Autodesk Inventor part; units mm, degrees
ref_plane "YZ Plane" through (0, 0, 0) normal (1, 0, 0) x (0, 1, 0)
ref_plane "XZ Plane" through (0, 0, 0) normal (0, 1, 0) x (-1, 0, 0)
ref_plane "XY Plane" through (0, 0, 0) normal (0, 0, 1) x (1, 0, 0)
sketch "Sketch1" plane through (0, 0, 0) normal (0, 0, 1) x (1, 0, 0)
  line L0 (0, 0) -> (15.24, 0)
  line L1 (21.2852, 0) -> (21.2852, 12.5984)
  line L2 (21.2852, 12.5984) -> (0, 12.5984)
  line L3 (0, 12.5984) -> (0, 0)
  line L4 (15.24, 0) -> (15.24, -15.621)
  line L5 (15.24, -15.621) -> (21.2852, -15.621)
  line L6 (21.2852, -15.621) -> (21.2852, 0)
  line L7 (0, 0) -> (15.24, 0)
  dimension "d0" = 21.2852
  dimension "d1" = 12.5984
  dimension "d2" = 6.0452
  dimension "d3" = 15.621
extrude "Extrusion1" add sketch "Sketch1" along normal blind 1.4986
sketch "Sketch2" plane through (0, 0, 1.4986) normal (0, 0, 1) x (1, 0, 0)
  circle A0 centre (4.572, 6.5532) radius 1.9558
  line L0 (21.2852, 12.5984) -> (0, 12.5984)
  line L1 (0, 12.5984) -> (0, 0)
  circle A1 centre (18.2626, 6.5532) radius 1.9558
  dimension "d6" = 3.9116
  dimension "d7" = 6.0452
  dimension "d8" = 4.572
  dimension "d11" = 13.6906
extrude "Extrusion2" cut sketch "Sketch2" against normal blind 25.4
sketch "Sketch3" plane through (0, 0, 1.4986) normal (0, 0, 1) x (1, 0, 0)
  circle A0 centre (18.2626, -11.6332) radius 1.4478
  line L0 (15.24, -15.621) -> (21.2852, -15.621)
  line L1 (15.24, 0) -> (15.24, -15.621)
  circle A1 centre (18.2626, -7.6708) radius 1.4478
  line L2 (16.8148, -7.6708) -> (18.2626, -7.6708)
  line L3 (19.7104, -11.6332) -> (17.1196, -11.6332)
  point P0 (0, 0)
  dimension "d18" = 2.8956
  dimension "d19" = 3.9878
  dimension "d20" = 3.0226
  dimension "d26" = 3.9624
extrude "Extrusion4" cut sketch "Sketch3" against normal blind 25.4
sketch "Sketch6" plane through (0, 0, 1.4986) normal (0, 0, 1) x (1, 0, 0)
  circle A0 centre (18.2626, -7.6708) radius 1.4478
  circle A1 centre (18.2626, -11.6332) radius 1.4478
  line L0 (16.8148, -7.6708) -> (19.7104, -7.6708)
  line L1 (19.7104, -7.6708) -> (19.7104, -11.6332)
  line L2 (19.7104, -11.6332) -> (16.8148, -11.6332)
  line L3 (16.8148, -11.6332) -> (16.8148, -7.6708)
  point P0 (0, 0)
extrude "Extrusion5" cut sketch "Sketch6" against normal blind 25.4 contours L1 A1 L3 A0 | A0 L0 | L2 A1 picked at (18.2044, -8.1499) picked at (18.4337, -11.182)
sketch "Sketch17" plane through (0, 0, 0) normal (0, 0, -1) x (-1, 0, 0)
  line L0 (-21.2852, -15.621) -> (-21.2852, 12.5984)
  line L1 (-21.2852, 0) -> (-15.349, 0)
  point P0 (0, 0)
bend part "Bend Part3" radius 1.4986 angle 90 line through (21.2852, 0, 0) along (-1, 0, 0) centre toward (0, 0, -1) moving side (0, -1, 0) both sides no
equation "\"BendRadius\" = Thickness"
equation "\"BendReliefWidth\" = Thickness"
equation "\"BendReliefDepth\" = 0.5 * Thickness"
equation "\"CornerReliefSize\" = 4 * Thickness"
equation "\"MinimumRemnant\" = 2 * Thickness"
equation "\"TransitionRadius\" = BendRadius"
equation "\"JacobiRadiusSize\" = Thickness"
equation "\"GapSize\" = Thickness"
properties part number "dsub37bracket_redraw"
CAD build for the part. Positions are in the model's coordinates, mm. A direction names the side the tool comes from. Coordinates: 2 decimals unless noted, no trailing zeros. Loops run counter-clockwise (first coordinate to the right, second up) from the corner with the lowest first, then second, coordinate; pieces in that order, holes last. Notation, with made-up numbers: (-23.5, 82) - (15.5, 82) arc R17 ccw to (15.5, 106) - close; hole circle Ø4 at (-8.5, -12.5). An arc over 180 degrees is marked (long way). Write item = value, one per line. Start each with the question number.
Q1. Pull direction Z, two halves, no side cores. Call faces 5 (the cylindrical face through (18.231, -2.258, -12.225)), 6 (the flat face through (0, 6, 1)), 7 (the flat face through (10, 6, 0)), 8 (the flat face through (10, 6, 1.499)): pulls with the +Z half, pulls with the -Z half, needs draft (parallel to the pull), parting line crosses it, or undercut.
Q2. Cut at C-C, the plane y = 5.75. List the corners of the cut face in (x, z), then the cut area to 3 significant figures.
Q3. Cut at A-A, the plane z = -8. List the corners of the cut face in (x, y).
Q4. Flat gauge pins, fed straight in: pin 1 Ø5 at (x, y) = (4.57, 6.55) entering from -Z; pin 2 Ø5 at (x, z) = (8, -2) entering from -Y; pin 3 Ø1.5 at (y, z) = (-1, -6) entering from -X. Where does each tip first touch, or does it go through?
Q5. Drill centre lines: L1, parallel to Z at x = 16, y = 1; L2, parallel to Y at x = 19.5, z = -13.25; L3, parallel to X at y = 7, z = 0.75. Where is each one in solid material? Low to high.
Q6. Cut at B-B, the plane x = 18.5. List the corners of the cut face in (y, z).
Q7. Cut at D-D, the plane x = 3.75. List the corners of the cut face in (y, z), then the cut area to 3 significant figures.
Q8. Which spindle directions (+Z, -Z, +X, -X, +Y, -Y) get a long thin tool onto all of the face, cutting with end or side? Do faces 1 (the flat face through (16, -2.997, -8)), 2 (the cylindrical face through (18.294, -2.258, -5.368)), 3 (the flat face through (8, 0, 1)), 4 (the flat face through (16, -1.499, -8)). Say none if no direction does.
Computed:
q1.face_5 = undercut
q1.face_6 = needs draft
q1.face_7 = pulls with the -Z half
q1.face_8 = pulls with the +Z half
q2.outline = (0, 0) - (2.79, 0) - (2.79, 1.5) - (0, 1.5) - close; (6.36, 0) - (16.48, 0) - (16.48, 1.5) - (6.36, 1.5) - close; (20.05, 0) - (21.29, 0) - (21.29, 1.5) - (20.05, 1.5) - close
q2.area = 21.2 mm²
q3.outline = (15.24, -3) - (16.81, -3) - (16.81, -1.5) - (15.24, -1.5) - close; (19.71, -3) - (21.29, -3) - (21.29, -1.5) - (19.71, -1.5) - close
q4.pin_1 = 0
q4.pin_2 = 0
q4.pin_3 = 15.24
q5.L1 = 0 to 1.5
q5.L2 = -3 to -1.5
q5.L3 = 0 to 2.67, 6.48 to 16.36, 20.17 to 21.29
q6.outline = (-3, -14.77) - (-1.5, -14.77) - (-1.5, -12.21) - (-3, -12.21) - close; (-3, -5.39) - (-1.5, -5.39) - (-1.5, -1.5) arc R1.5 cw to (0, 0) - (4.61, 0) - (4.61, 1.5) - (0, 1.5) arc R3 ccw to (-3, -1.5) - close; (8.49, 0) - (12.6, 0) - (12.6, 1.5) - (8.49, 1.5) - close
q7.outline = (0, 0) - (4.78, 0) - (4.78, 1.5) - (0, 1.5) - close; (8.33, 0) - (12.6, 0) - (12.6, 1.5) - (8.33, 1.5) - close
q7.area = 13.6 mm²
q8.face_1 = +Z, -Z, +X, -X, -Y
q8.face_2 = +Y, -Y
q8.face_3 = +Z, -Z, -X, -Y
q8.face_4 = -Z, +X, -X, +Y
